Part print with two shaded views. Sizes in mm from the minimum x, y, z corner. Round coordinates to 2 decimals unless told otherwise and drop trailing zeros. Write each loop counter-clockwise with the first axis right and the second up, starting at its lowest first coordinate (ties: lowest second). Pieces come first, ordered by that corner, then holes. Notation, with made-up numbers: (-21, 81) - (7, 81) arc R15 cw to (7, 88) - close; hole circle Ø11 at (85, 66.25). An arc over 180 degrees is marked (long way). Use one line per item in the form item = value. Start each with the question number.
Item 1: Band-saw the part on C-C, the plane z = 30. List the corners of the cut face in (x, y), and give its area (3 significant figures).
Item 2: Band-saw the part on A-A, the plane z = 9.35. List the corners of the cut face in (x, y).
Item 3: Band-saw the part on D-D, the plane x = 139.5. List the corners of the cut face in (y, z), and give its area (3 significant figures).
Item 4: Band-saw the part on B-B, the plane x = 100.33. List the corners of the cut face in (y, z).
Item 5: Pin check, flat tips, straight feed: pin 1 (2 mm diameter, centred on x = 128.27, z = 72.85, fed in from +Y); pin 2 (4.5 mm diameter, centred on x = 88.9, z = 1.905, fed in from -Y); pin 3 (1.5 mm diameter, centred on x = 65.5, y = 2, fed in from +Z). Stop position of each tip, or through.
Item 6: Drill centre lines: L1, parallel to X at y = 2.05, z = 72.85; L2, parallel to Z at x = 38, y = 2.95 (1 decimal); L3, parallel to X at y = 0.45, z = 46.5. Where is each one in solid material? Low to high.
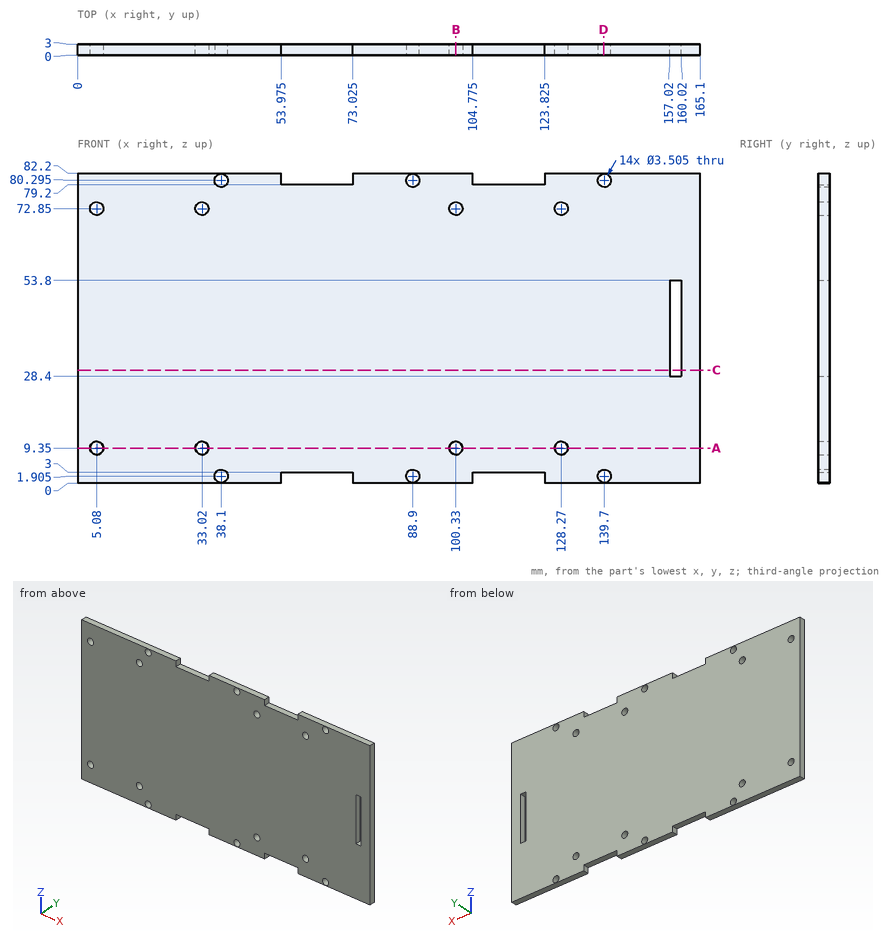
Determined:
q1.outline = (0, 0) - (157.02, 0) - (157.02, 3) - (0, 3) - close; (160.02, 0) - (165.1, 0) - (165.1, 3) - (160.02, 3) - close
q1.area = 486 mm²
q2.outline = (0, 0) - (3.33, 0) - (3.33, 3) - (0, 3) - close; (6.83, 0) - (31.27, 0) - (31.27, 3) - (6.83, 3) - close; (34.77, 0) - (98.58, 0) - (98.58, 3) - (34.77, 3) - close; (102.08, 0) - (126.52, 0) - (126.52, 3) - (102.08, 3) - close; (130.02, 0) - (165.1, 0) - (165.1, 3) - (130.02, 3) - close
q3.outline = (0, 0) - (3, 0) - (3, 0.16) - (0, 0.16) - close; (0, 3.65) - (3, 3.65) - (3, 78.55) - (0, 78.55) - close; (0, 82.04) - (3, 82.04) - (3, 82.2) - (0, 82.2) - close
q3.area = 226 mm²
q4.outline = (0, 0) - (3, 0) - (3, 7.6) - (0, 7.6) - close; (0, 11.1) - (3, 11.1) - (3, 71.1) - (0, 71.1) - close; (0, 74.6) - (3, 74.6) - (3, 82.2) - (0, 82.2) - close
q5.pin_1 = through
q5.pin_2 = 0
q5.pin_3 = 79.2
q6.L1 = 0 to 3.33, 6.83 to 31.27, 34.77 to 98.58, 102.08 to 126.52, 130.02 to 165.1
q6.L2 = 0 to 0.2, 3.7 to 78.5, 82 to 82.2
q6.L3 = 0 to 157.02, 160.02 to 165.1
